Study the drawing (mm; zero at the part's minimum x, y, z) and answer. Give positions to 0.01 mm unless a question says otherwise; leave off trailing zeros. Order: outer loops, then holes, each group sorted by start corner. A loop starts at its lowest first (then second) coordinate and runs counter-clockwise, first axis right, second up. Notation, with made-up numbers: (70, 70) - (110, 70) arc R17 cw to (110, 95) - close; hole circle Ø1 at (35.5, 32.5). An arc over 180 degrees is marked (long way). Use CSV: the item, a comma, the result in double quotes.
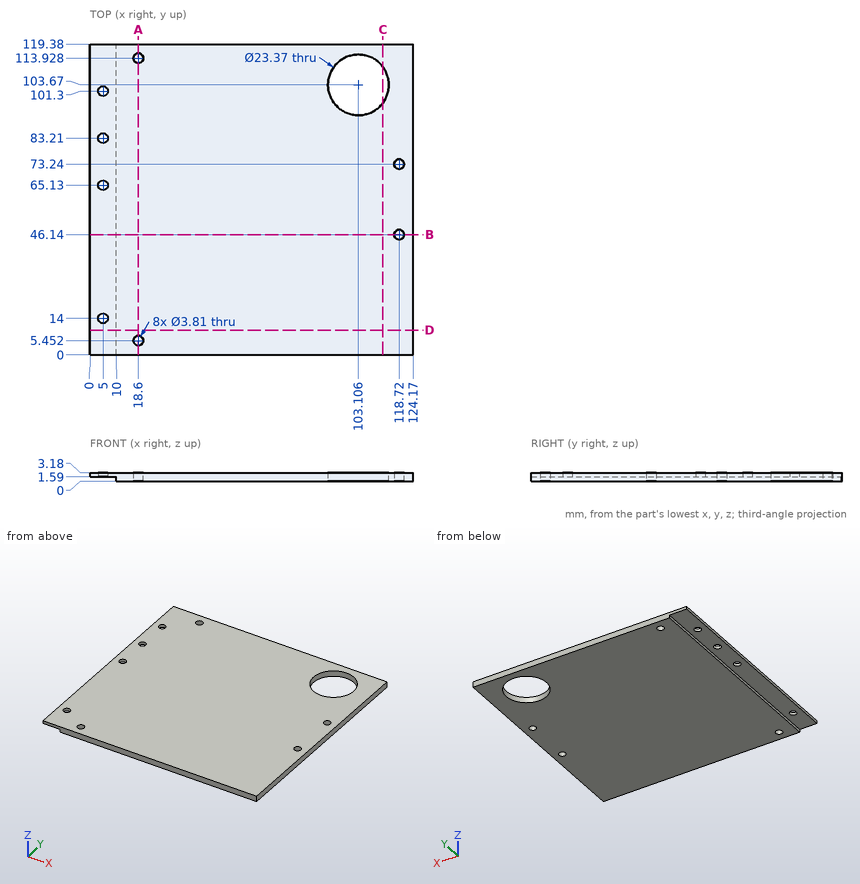
Item 1: Each of these flat-tipped pins is pushed along its axis until it touches: pin 1 (3.5 mm diameter, centred on x = 5, y = 14, fed in from +Z); pin 2 (5 mm diameter, centred on x = 4.5, y = 88.5, fed in from -Z). Where does it stop, or does it pass through?
Taken from the geometry:
pin 1,"through"
pin 2,"z = 1.59"
Item 2: The part is cut by section B-B (y = 46.14). Give the vertices of the cut face in (x, z) (3 decimals), and give its area (3 significant figures).
Taken from the geometry:
outline,"(0, 1.59) - (10, 1.59) - (10, 0) - (116.815, 0) - (116.815, 3.18) - (0, 3.18) - close; (120.625, 0) - (124.17, 0) - (124.17, 3.18) - (120.625, 3.18) - close"
area,"367 mm^2"
Item 3: Find the intervals of material crossed by line 1 along Y through (x, z) = (118.72, 1.05) (3 decimals); line 2 along Y through (x, z) = (18.6, 0.95); line 3 along X through (y, z) = (103.67, 1.25), in increasing order.
Taken from the geometry:
line 1,"0 to 44.235, 48.045 to 71.335, 75.145 to 119.38"
line 2,"0 to 3.55, 7.36 to 112.02, 115.83 to 119.38"
line 3,"10 to 91.42, 114.79 to 124.17"
Item 4: The part is cut by section A-A (x = 18.6). Give the vertices of the cut face in (y, z).
Taken from the geometry:
outline,"(0, 0) - (3.55, 0) - (3.55, 3.18) - (0, 3.18) - close; (7.36, 0) - (112.02, 0) - (112.02, 3.18) - (7.36, 3.18) - close; (115.83, 0) - (119.38, 0) - (119.38, 3.18) - (115.83, 3.18) - close"
Item 5: The part is cut by section C-C (x = 112.5). Give the vertices of the cut face in (y, z), and give its area (3 significant figures).
Taken from the geometry:
outline,"(0, 0) - (96.72, 0) - (96.72, 3.18) - (0, 3.18) - close; (110.62, 0) - (119.38, 0) - (119.38, 3.18) - (110.62, 3.18) - close"
area,"335 mm^2"
Item 6: The part is cut by section D-D (y = 9.5). Give the vertices of the cut face in (x, z).
Taken from the geometry:
outline,"(0, 1.59) - (10, 1.59) - (10, 0) - (124.17, 0) - (124.17, 3.18) - (0, 3.18) - close"
